The model under review builds one solid part; all positions refer to its coordinate system, in mm. Face numbers are marked on the shaded views. A direction names the side the tool comes from. Coordinates: 2 decimals unless noted, no trailing zeros.
1) Mouldability with a two-part tool opening along Z and no side actions: class the marked faces 1 and 2 as released by +Z, released by -Z, zero draft, split by the parting line, or undercut.
2) Machinability: for the marked faces 3 and 4, which of the approach directions +Z, -Z, +X, -X, +Y, -Y give a long, thin tool a straight path to every point of the face, cutting with its end or side? Answer none if there is none.
3) For line 1 (Z direction, x = -9, y = 0); line 2 (Z direction, x = 11.5, y = 215.5); line 3 (Z direction, x = 2.75, y = 0), list the stretches that pass through material, from the lowest coordinate up.
4) For P1, Ø5, axis at x = -14, y = -342.5, coming from the -Z side; P2, Ø3, axis at x = 29, z = 182.5, coming from the +Y side; P3, Ø8, axis at x = 15, y = 271.5, coming from the +Z side, all flat-tipped, find the tip position at first contact; note any pin that passes through.
from build123d import *
from build123d.topology import SkipClean

# Parameters (mm, degrees)
CUT_EXTRUDE3_DEPTH = 10
CIRPATTERN1_COUNT  = 9


with BuildPart() as part:
    # Sketch1 → Revolve1 (revolve)
    with BuildSketch(Plane.XY, mode=Mode.PRIVATE) as revolve1_sk:
        Polygon((-40, 100), (-40, 0), (40, 0), (40, 430), (20.490381057, 449.509618943), (0, 455), (-20, 455), (-20, 410), (10, 410), (10, 100), (-20, 100), align=None)
    revolve(revolve1_sk.sketch.rotate(Axis((-40, 0, 0), (1, 0, 0)), 180), axis=Axis((-40, 0, 0), (1, 0, 0)))

    # Sketch2 → Cut-Extrude3 (cut)
    with SkipClean():  # the faces are left unmerged after this step: merging them gives an invalid solid
        with BuildSketch(Plane.ZY.offset(-10)):
            with BuildLine():
                Line((20, 105.830052443), (20, 398.873413504))
                ThreePointArc((20, 398.873413504), (23.199264746, 406.204852653), (30.75, 408.845248841))
                ThreePointArc((30.75, 408.845248841), (109.265252373, 395.172246778), (183.651957914, 366.567808672))
                ThreePointArc((183.651957914, 366.567808672), (215.530603819, 325.085308606), (202.738728221, 274.356482529))
                Line((202.738728221, 274.356482529), (51.709811994, 94.367229029))
                ThreePointArc((51.709811994, 94.367229029), (46.332346285, 91.059191807), (40.044879602, 91.631913751))
                ThreePointArc((40.044879602, 91.631913751), (33.736520206, 94.137384733), (27.272727273, 96.209138584))
                ThreePointArc((27.272727273, 96.209138584), (22.022759648, 99.799825551), (20, 105.830052443))
            make_face()
        cut_extrude3 = extrude(amount=-CUT_EXTRUDE3_DEPTH, mode=Mode.SUBTRACT)

    # CirPattern1: Cut-Extrude3 ×9 about axis
    with SkipClean():  # the faces are left unmerged after this step: merging them gives an invalid solid
        cirpattern1_axis = Axis((0, 0, 0), (1, 0, 0))
        for i in range(1, CIRPATTERN1_COUNT):
            add(cut_extrude3.rotate(cirpattern1_axis, i * 360 / CIRPATTERN1_COUNT), mode=Mode.SUBTRACT)


solid = part.part
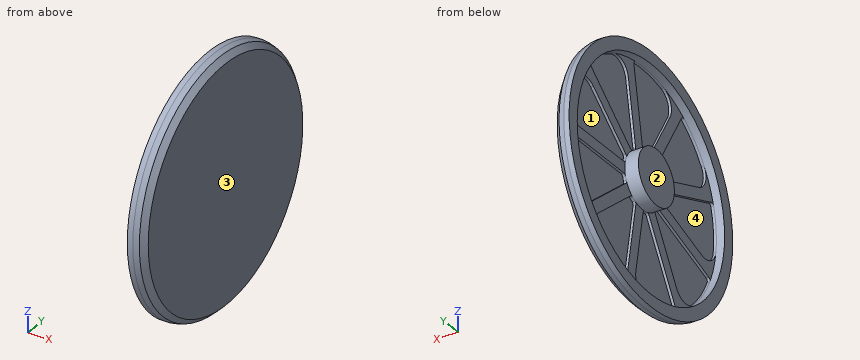
Geometry results:
1. face 1: undercut
1. face 2: zero draft
2. face 3: +Z, -Z, +X, +Y, -Y
2. face 4: -X
3. line 1: z = -455 to -410, -100 to 100, 410 to 455
3. line 2: z = -397.23 to -348.8, -208.3 to -154.72, -21.05 to 20, 153.35 to 206.93, 348.8 to 397.23
3. line 3: z = -454.26 to -410, -100 to 100, 410 to 454.26
4. P1: stops at z = -302.37
4. P2: stops at y = 403.25
4. P3: stops at z = 363.37
